Read the model definition and answer for the solid it produces. Units are mm, in the model's axes. A direction names the side the tool comes from. Give positions to 0.01 mm unless a question says otherwise; leave off trailing zeros. Write each loop counter-clockwise with the first axis right and the second up, starting at its lowest first coordinate (ties: lowest second). Pieces come first, ordered by that corner, then holes. Notation, with made-up numbers: (-29, 3.5) -> (30, 3.5) arc R9 ccw to (30, 11.5) -> close; hole circle Ø7 at (24, 82). An arc over 180 degrees is marked (long way). Write item = value, one per line.
from build123d import *

# Parameters (mm, degrees)
SKETCH1_R           = 5
BOSS_EXTRUDE1_DEPTH = 9.5
BOSS_EXTRUDE2_DEPTH = 30
SKETCH2_R           = 5
CUT_EXTRUDE1_DEPTH  = 21
FILLET1_R           = 10
FILLET2_R           = 5


with BuildPart() as part:
    # Sketch1 → Boss-Extrude1 (new body, symmetric)
    with BuildSketch(Plane(origin=(0, 0, 0), x_dir=(1, 0, 0), z_dir=(0, 1, 0))):
        with BuildLine():
            Line((10.5, 10), (0, 10))
            ThreePointArc((0, 10), (-10, 0), (0, -10))
            Line((0, -10), (10.5, -10))
            Line((10.5, -10), (10.5, 10))
        make_face()
        Circle(SKETCH1_R, mode=Mode.SUBTRACT)
    extrude(amount=BOSS_EXTRUDE1_DEPTH, both=True)

    # Sketch1<3> → Boss-Extrude2 (add, symmetric)
    with BuildSketch(Plane(origin=(0, 0, 0), x_dir=(1, 0, 0), z_dir=(0, 1, 0))):
        Polygon((40.5, 10), (10.5, 10), (10.5, -10), (40.5, -10), (40.5, -5), (20.5, -5), (20.5, 5), (40.5, 5), align=None)
    extrude(amount=BOSS_EXTRUDE2_DEPTH, both=True)

    # Sketch2 → Cut-Extrude1 (cut, through all)
    with BuildSketch(Plane.XY.offset(10)):
        with Locations((30, 20)):
            Circle(SKETCH2_R)
        with Locations((30, -20)):
            Circle(SKETCH2_R)
    extrude(amount=-CUT_EXTRUDE1_DEPTH, mode=Mode.SUBTRACT)

    # Fillet1
    fillet1_edges = [part.edges().sort_by_distance(p)[0] for p in [
        (40.5, -30, -7.5),
        (40.5, -30, 7.5),
        (40.5, 30, -7.5),
        (40.5, 30, 7.5),
    ]]
    fillet(fillet1_edges, radius=FILLET1_R)

    # Fillet2
    fillet2_edges = [part.edges().sort_by_distance(p)[0] for p in [
        (10.5, 19.75, -10),
        (10.5, -19.75, -10),
        (10.5, 19.75, 10),
        (10.5, -19.75, 10),
    ]]
    fillet(fillet2_edges, radius=FILLET2_R)


solid = part.part
(1) A tool of negligible diameter and unlimited length cuts with its end or side. For faces 1 (the flat face through (10.5, -20, 0)), 2 (the flat face through (30, 0, -5)), 3 (the cylindrical face through (12, 19.89, -8.57)), 4 (the flat face through (10.5, 20, 0)), from which of +Z, -Z, +X, -X, +Y, -Y can it reach the whole face along a straight path? Write none if from no direction.
Checks:
face_1 = +Z, -Z, -X, -Y
face_2 = +X, +Y, -Y
face_3 = -Z, -X, +Y
face_4 = +Z, -Z, -X, +Y
(2) The part is cut by section A-A on y = -3. Determine the outline of the cut face in (x, z), plus the area to 3 significant figures.
Checks:
outline = (0, -10) -> (40.5, -10) -> (40.5, -5) -> (20.5, -5) -> (20.5, 5) -> (40.5, 5) -> (40.5, 10) -> (0, 10) arc R10 ccw to start; hole circle Ø10 at (0, 0)
area = 689 mm²
(3) Given P1, Ø6, axis at x = 30, y = 20, coming from the +Z side; P2, Ø8, axis at y = 9.5, z = 1, coming from the -X side; P3, Ø3, axis at y = 13.5, z = -2, coming from the +X side; P4, Ø6, axis at x = 3, z = 1.5, coming from the +Y side, each flat-ended and moving along its own axis, determine where each tip first touches the part or whether it passes through.
Checks:
P1 = through
P2 = -10
P3 = 20.5
P4 = 9.5
(4) The part is cut by section C-C on z = 8.5. Determine the outline of the cut face in (x, y), plus the area to 3 significant figures.
Checks:
outline = (-5.27, -9.5) -> (11.93, -9.5) -> (11.93, -30) -> (30.5, -30) arc R10 ccw to (40.5, -20) -> (40.5, 20) arc R10 ccw to (30.5, 30) -> (11.93, 30) -> (11.93, 9.5) -> (-5.27, 9.5) -> close; hole circle Ø10 at (30, -20); hole circle Ø10 at (30, 20)
area = 1,840 mm²
(5) The part is cut by section D-D on z = -3.5. Determine the outline of the cut face in (x, y), plus the area to 3 significant figures.
Checks:
outline = (-9.37, -9.5) -> (-3.57, -9.5) -> (-3.57, 9.5) -> (-9.37, 9.5) -> close; (3.57, -9.5) -> (10.5, -9.5) -> (10.5, -30) -> (20.5, -30) -> (20.5, 30) -> (10.5, 30) -> (10.5, 9.5) -> (3.57, 9.5) -> close
area = 842 mm²
(6) The part is cut by section B-B on x = 32. Determine the outline of the cut face in (y, z), plus the area to 3 significant figures.
Checks:
outline = (-29.89, -10) -> (-24.58, -10) -> (-24.58, -5) -> (-29.89, -5) -> close; (-29.89, 5) -> (-24.58, 5) -> (-24.58, 10) -> (-29.89, 10) -> close; (-15.42, -10) -> (15.42, -10) -> (15.42, -5) -> (-15.42, -5) -> close; (-15.42, 5) -> (15.42, 5) -> (15.42, 10) -> (-15.42, 10) -> close; (24.58, -10) -> (29.89, -10) -> (29.89, -5) -> (24.58, -5) -> close; (24.58, 5) -> (29.89, 5) -> (29.89, 10) -> (24.58, 10) -> close
area = 414 mm²
(7) Consider L1, parallel to Y at x = 30, z = -6.95; L2, parallel to Z at x = 21.5, y = 19; L3, parallel to X at y = 2.25, z = 0. Determine where each line is inside the solid, lowest interval first.
Checks:
L1 = -30 to -25, -15 to 15, 25 to 30
L2 = -10 to -5, 5 to 10
L3 = -10 to -5, 5 to 20.5
(8) For a pull along Y with two mould halves and no side action, classify faces 5 (the flat face through (40.5, 0, 8)), 6 (the cylindrical face through (26, 17, 8)), 7 (the cylindrical face through (37.65, 26.99, -7.54)), 8 (the cylindrical face through (37.49, -27.15, 7.46)) as released by +Y, released by -Y, zero draft, split by the parting line, or undercut.
Checks:
face_5 = zero draft
face_6 = undercut
face_7 = released by +Y
face_8 = released by -Y
